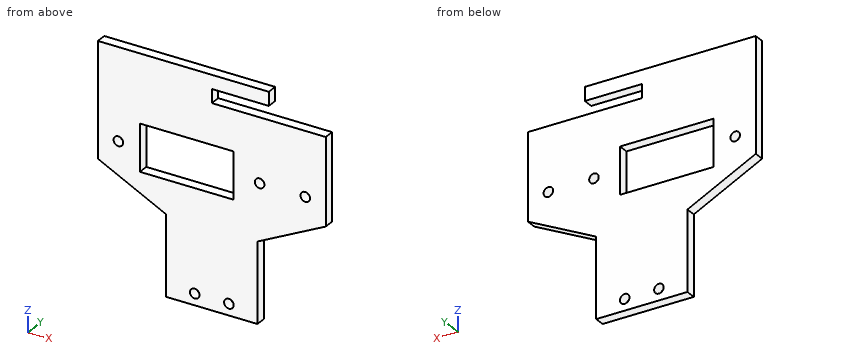
```python
from build123d import *

# Parameters (mm, degrees)
SKETCH1_R           = 2.1
BOSS_EXTRUDE1_DEPTH = 4.5
SKETCH2_W           = 41.1
SKETCH2_H           = 20.5
CUT_EXTRUDE1_DEPTH  = 10
CUT_EXTRUDE2_DEPTH  = 10
SKETCH4_R           = 2.1
CUT_EXTRUDE3_DEPTH  = 10


with BuildPart() as part:
    # Sketch1 → Boss-Extrude1 (new body)
    with BuildSketch(Plane(origin=(0, 0, 0), x_dir=(1, 0, 0), z_dir=(0, 1, 0))):
        Polygon((20, 40), (50, 25), (50, -25), (-50, -25), (-50, 25), (-20, 40), (-20, 75), (20, 75), align=None)
        with Locations((-41, 15)):
            Circle(SKETCH1_R, mode=Mode.SUBTRACT)
        with Locations((41, 15)):
            Circle(SKETCH1_R, mode=Mode.SUBTRACT)
        with Locations((-21, 15)):
            Circle(SKETCH1_R, mode=Mode.SUBTRACT)
        with Locations((21, 15)):
            Circle(SKETCH1_R, mode=Mode.SUBTRACT)
    extrude(amount=BOSS_EXTRUDE1_DEPTH)

    # Sketch2 → Cut-Extrude1 (cut)
    with BuildSketch(Plane.XZ):
        with Locations((-11, -15)):
            Rectangle(SKETCH2_W, SKETCH2_H)
    extrude(amount=-CUT_EXTRUDE1_DEPTH, mode=Mode.SUBTRACT)

    # Sketch3 → Cut-Extrude2 (cut)
    with BuildSketch(Plane.XZ):
        Polygon((0, 19), (25, 19), (25, 28.725277581), (50, 28.725277581), (50, 19), (50, 13), (0, 13), align=None)
    extrude(amount=-CUT_EXTRUDE2_DEPTH, mode=Mode.SUBTRACT)

    # Sketch4 → Cut-Extrude3 (cut)
    with BuildSketch(Plane(origin=(0, 4.5, 0), x_dir=(1, 0, 0), z_dir=(0, 1, 0))):
        with Locations((7.5, 70)):
            Circle(SKETCH4_R)
        with Locations((-7.5, 70)):
            Circle(SKETCH4_R)
    extrude(amount=-CUT_EXTRUDE3_DEPTH, mode=Mode.SUBTRACT)


solid = part.part
```
Could you check a few things on this model? Use its own coordinates, in mm. Coordinates: 2 decimals unless noted, no trailing zeros. Write each loop counter-clockwise with the first axis right and the second up, starting at its lowest first coordinate (ties: lowest second). Pieces come first, ordered by that corner, then holes. Notation, with made-up numbers: (32, -1.75) - (62, -1.75) arc R17 ccw to (62, 29.25) - close; hole circle Ø7 at (-36.5, 41.5). An arc over 180 degrees is marked (long way). Use a Markdown table: item, result.
Q1. Imagine slicing it at C-C (y = 1.25). List the corners of the cut face in (x, z) for me, and give its area (3 significant figures).
Geometry check:
| item | result |
|---|---|
| outline | (-50, -25) - (-20, -40) - (-20, -75) - (20, -75) - (20, -40) - (50, -25) - (50, 13) - (0, 13) - (0, 19) - (25, 19) - (25, 25) - (-50, 25) - close; hole circle Ø4.2 at (-41, -15); hole (-31.55, -25.25) - (9.55, -25.25) - (9.55, -4.75) - (-31.55, -4.75) - close; hole circle Ø4.2 at (-7.5, -70); hole circle Ø4.2 at (7.5, -70); hole circle Ø4.2 at (21, -15); hole circle Ø4.2 at (41, -15) |
| area | 6,090 mm2 |
Q2. I'm going to push flat-ended pins straight in: pin 1 Ø1.3 at (y, z) = (2.5, 21.5) entering from +X; pin 2 Ø2 at (y, z) = (1, -55) entering from -X; pin 3 Ø1.3 at (y, z) = (2.5, 16.5) entering from +X. Where does each tip first touch, or does it pass through?
Geometry check:
| item | result |
|---|---|
| pin 1 | stops at x = 25 |
| pin 2 | stops at x = -20 |
| pin 3 | stops at x = 0 |
Q3. Imagine slicing it at A-A (x = -7.5). List the corners of the cut face in (y, z) for me, and give its area (3 significant figures).
Geometry check:
| item | result |
|---|---|
| outline | (0, -75) - (4.5, -75) - (4.5, -72.1) - (0, -72.1) - close; (0, -67.9) - (4.5, -67.9) - (4.5, -25.25) - (0, -25.25) - close; (0, -4.75) - (4.5, -4.75) - (4.5, 25) - (0, 25) - close |
| area | 339 mm2 |
Q4. Please list where these lines run through material, in increasing order: L1, parallel to X at y = 2.95, z = -15; L2, parallel to X at y = 1.75, z = -70; L3, parallel to Z at x = 0.5, y = 3.4.
Geometry check:
| item | result |
|---|---|
| L1 | x = -50 to -43.1, -38.9 to -31.55, 9.55 to 18.9, 23.1 to 38.9, 43.1 to 50 |
| L2 | x = -20 to -9.6, -5.4 to 5.4, 9.6 to 20 |
| L3 | z = -75 to -25.25, -4.75 to 13, 19 to 25 |
Q5. Imagine slicing it at D-D (z = -10.5). List the corners of the cut face in (x, y) for me.
Geometry check:
| item | result |
|---|---|
| outline | (-50, 0) - (-31.55, 0) - (-31.55, 4.5) - (-50, 4.5) - close; (9.55, 0) - (50, 0) - (50, 4.5) - (9.55, 4.5) - close |
Q6. Imagine slicing it at B-B (x = 41). List the corners of the cut face in (y, z) for me.
Geometry check:
| item | result |
|---|---|
| outline | (0, -29.5) - (4.5, -29.5) - (4.5, -17.1) - (0, -17.1) - close; (0, -12.9) - (4.5, -12.9) - (4.5, 13) - (0, 13) - close |
